```python
from build123d import *

# Parameters (mm, degrees)
F0_W           = 101.6
F0_H           = 101.6
F1_DEPTH       = 12.7
F3_DEPTH       = 6.35
F8_D           = 4.0386
F8_DEPTH       = 15.08125
F8_TIP         = 1.213317848
F8_ON_F7_D     = 4.0386
F8_ON_F7_DEPTH = 15.08125
F8_ON_F7_TIP   = 1.213317848
F8_ON_F6_D     = 4.0386
F8_ON_F6_DEPTH = 15.08125
F8_ON_F6_TIP   = 1.213317848
F8_ON_F5_D     = 4.0386
F8_ON_F5_DEPTH = 15.08125
F8_ON_F5_TIP   = 1.213317848


with BuildPart() as f1:
    # F0 (on Top) → F1 (new body)
    with BuildSketch(Plane.XY):
        Rectangle(F0_W, F0_H)
    extrude(amount=F1_DEPTH)

    # F2 (on face) → F3 (cut)
    with BuildSketch(Plane(origin=(0, 0, 0), x_dir=(1, 0, 0), z_dir=(0, 0, -1))):
        with BuildLine():
            Line((-12.1741207811, 16.6642488417), (0, 4.4901280605))
            Line((0, 4.4901280605), (12.1741207811, 16.6642488417))
            ThreePointArc((12.1741207811, 16.6642488417), (0, 20.6375), (-12.1741207811, 16.6642488417))
        make_face()
        with BuildLine():
            Line((39.9598719395, 44.45), (-39.9598719395, 44.45))
            Line((-39.9598719395, 44.45), (-16.705457483, 21.1955855435))
            ThreePointArc((-16.705457483, 21.1955855435), (0, 26.9875), (16.705457483, 21.1955855435))
            Line((16.705457483, 21.1955855435), (39.9598719395, 44.45))
        make_face()
        with BuildLine():
            Line((-44.45, 39.9598719395), (-44.45, -39.9598719395))
            Line((-44.45, -39.9598719395), (-21.1955855435, -16.705457483))
            ThreePointArc((-21.1955855435, -16.705457483), (-26.9875, 0), (-21.1955855435, 16.705457483))
            Line((-21.1955855435, 16.705457483), (-44.45, 39.9598719395))
        make_face()
        with BuildLine():
            Line((-16.6642488417, -12.1741207811), (-4.4901280605, 0))
            Line((-4.4901280605, 0), (-16.6642488417, 12.1741207811))
            ThreePointArc((-16.6642488417, 12.1741207811), (-20.6375, 0), (-16.6642488417, -12.1741207811))
        make_face()
        with BuildLine():
            Line((-39.9598719395, -44.45), (39.9598719395, -44.45))
            Line((39.9598719395, -44.45), (16.705457483, -21.1955855435))
            ThreePointArc((16.705457483, -21.1955855435), (0, -26.9875), (-16.705457483, -21.1955855435))
            Line((-16.705457483, -21.1955855435), (-39.9598719395, -44.45))
        make_face()
        with BuildLine():
            Line((12.1741207811, -16.6642488417), (0, -4.4901280605))
            Line((0, -4.4901280605), (-12.1741207811, -16.6642488417))
            ThreePointArc((-12.1741207811, -16.6642488417), (0, -20.6375), (12.1741207811, -16.6642488417))
        make_face()
        with BuildLine():
            Line((44.45, -39.9598719395), (44.45, 39.9598719395))
            Line((44.45, 39.9598719395), (21.1955855435, 16.705457483))
            ThreePointArc((21.1955855435, 16.705457483), (26.9875, 0), (21.1955855435, -16.705457483))
            Line((21.1955855435, -16.705457483), (44.45, -39.9598719395))
        make_face()
        with BuildLine():
            Line((16.6642488417, 12.1741207811), (4.4901280605, 0))
            Line((4.4901280605, 0), (16.6642488417, -12.1741207811))
            ThreePointArc((16.6642488417, -12.1741207811), (20.6375, 0), (16.6642488417, 12.1741207811))
        make_face()
    extrude(amount=-F3_DEPTH, mode=Mode.SUBTRACT)

    # F8
    with Locations(Plane.XZ.offset(50.8)):
        with Locations((-16.9333333333, 6.35), (16.9333333333, 6.35)):
            Hole(F8_D / 2, depth=F8_DEPTH)
            with Locations((0, 0, -(F8_DEPTH + F8_TIP / 2))):  # 118° drill point
                Cone(0, F8_D / 2, F8_TIP, mode=Mode.SUBTRACT)

    # F8 on F7
    with Locations(Plane(origin=(-50.8, 0, 0), x_dir=(0, -1, 0), z_dir=(-1, 0, 0))):
        with Locations((16.9333333333, 6.35), (-16.9333333333, 6.35)):
            Hole(F8_ON_F7_D / 2, depth=F8_ON_F7_DEPTH)
            with Locations((0, 0, -(F8_ON_F7_DEPTH + F8_ON_F7_TIP / 2))):  # 118° drill point
                Cone(0, F8_ON_F7_D / 2, F8_ON_F7_TIP, mode=Mode.SUBTRACT)

    # F8 on F6
    with Locations(Plane(origin=(0, 50.8, 0), x_dir=(-1, 0, 0), z_dir=(0, 1, 0))):
        with Locations((16.9333333333, 6.35), (-16.9333333333, 6.35)):
            Hole(F8_ON_F6_D / 2, depth=F8_ON_F6_DEPTH)
            with Locations((0, 0, -(F8_ON_F6_DEPTH + F8_ON_F6_TIP / 2))):  # 118° drill point
                Cone(0, F8_ON_F6_D / 2, F8_ON_F6_TIP, mode=Mode.SUBTRACT)

    # F8 on F5
    with Locations(Plane.YZ.offset(50.8)):
        with Locations((16.9333333333, 6.35), (-16.9333333333, 6.35)):
            Hole(F8_ON_F5_D / 2, depth=F8_ON_F5_DEPTH)
            with Locations((0, 0, -(F8_ON_F5_DEPTH + F8_ON_F5_TIP / 2))):  # 118° drill point
                Cone(0, F8_ON_F5_D / 2, F8_ON_F5_TIP, mode=Mode.SUBTRACT)


solid = f1.part
```
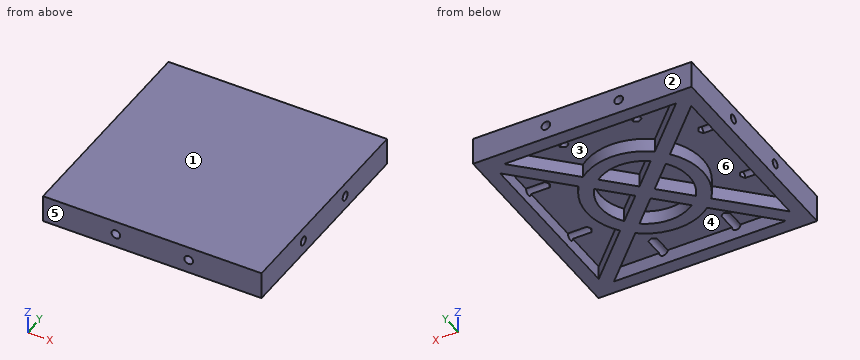
Geometry: final body of the model. Coordinates: model frame, mm. Face numbers are marked on the shaded views. A direction names the side the tool comes from. Coordinates: 2 decimals unless noted, no trailing zeros. Order: outer loops, then holes, each group sorted by start corner. A loop starts at its lowest first (then second) coordinate and runs counter-clockwise, first axis right, second up. Notation, with made-up numbers: (9.25, -34) -> (65.25, -34) arc R15 cw to (65.25, -9) -> close; hole circle Ø7 at (52.5, -2.5). An arc over 180 degrees is marked (long way). Write item = value, one per line.
(1) Cut plane A-A on z = 1.75. Count the separate pieces of the cut face and the enclosed holes in it, plus the area to 3 significant figures.
Solved:
separate_pieces = 1
enclosed_holes = 8
area = 4,720 mm²
(2) Pull-direction query (Y, two-part tool) for the marked faces 1, 2, 3 and 4; classes: pulls with the +Y half, pulls with the -Y half, needs draft (parallel to the pull), parting line crosses it, or undercut.
Solved:
face_1 = needs draft
face_2 = pulls with the +Y half
face_3 = undercut
face_4 = undercut
(3) Cut plane C-C on y = -3. Return loops of the section in (x, z), plus the area to 3 significant figures.
Solved:
outline = (-50.8, 0) -> (-44.45, 0) -> (-44.45, 6.35) -> (-26.82, 6.35) -> (-26.82, 0) -> (-20.42, 0) -> (-20.42, 6.35) -> (-7.49, 6.35) -> (-7.49, 0) -> (7.49, 0) -> (7.49, 6.35) -> (20.42, 6.35) -> (20.42, 0) -> (26.82, 0) -> (26.82, 6.35) -> (44.45, 6.35) -> (44.45, 0) -> (50.8, 0) -> (50.8, 12.7) -> (-50.8, 12.7) -> close
area = 902 mm²
(4) Line query: line 1 (X direction, y = 47.25, z = 6.35); line 2 (X direction, y = -39.5, z = 3). Output: solid intervals per line, ascending.
Solved:
line_1 = -50.8 to -18.95, -14.91 to 14.91, 18.95 to 50.8
line_2 = -50.8 to -44.45, -43.99 to -35.01, 35.01 to 43.99, 44.45 to 50.8
(5) Cut plane B-B on x = -33. Return loops of the section in (y, z).
Solved:
outline = (-50.8, 0) -> (-44.45, 0) -> (-44.45, 6.35) -> (-37.49, 6.35) -> (-37.49, 0) -> (-28.51, 0) -> (-28.51, 6.35) -> (28.51, 6.35) -> (28.51, 0) -> (37.49, 0) -> (37.49, 6.35) -> (44.45, 6.35) -> (44.45, 0) -> (50.8, 0) -> (50.8, 12.7) -> (-50.8, 12.7) -> close
(6) Access query for the marked faces 5 and 6. Directions: +Z, -Z, +X, -X, +Y, -Y. A direction counts if a zero-diameter tool reaches every point of the face in a straight line with its end or side. Return the directions, or none.
Solved:
face_5 = +Z, -Z, +X, -X, -Y
face_6 = -Z
(7) Pin query (flat end, axial travel): pin 1 Ø2.5 at (x, z) = (16.93, 6.35) entering from +Y; pin 2 Ø3 at (y, z) = (-16.93, 6.35) entering from -X; pin 3 Ø5 at (x, y) = (5, 16.5) entering from -Z. Return the tip coordinate at first contact, or that it passes through.
Solved:
pin_1 = 35.26
pin_2 = -35.41
pin_3 = 6.35
